Source: CAD feature listing. Evaluate the final solid. Frame: model axes, mm. Face numbers are marked on the shaded views. A direction names the side the tool comes from. Round coordinates to 2 decimals unless told otherwise and drop trailing zeros. Order: outer loops, then holes, each group sorted by start corner. A loop starts at its lowest first (then second) coordinate and runs counter-clockwise, first axis right, second up. Notation, with made-up numbers: (-31, 61.25) -> (4, 61.25) arc R22 cw to (4, 68.25) -> close; hole circle Ø6 at (-23, 38.25). An arc over 180 degrees is marked (long way). Answer as CSV lines item,"result".
from build123d import *

# Parameters (mm, degrees)
SKETCH1_W               = 40
SKETCH1_H               = 32
BOSS_EXTRUDE1_DEPTH     = 7
SKETCH2_R               = 14.05
CUT_EXTRUDE1_DEPTH      = 6
SKETCH3_R               = 8.7
CUT_EXTRUDE2_DEPTH      = 6
SKETCH4_R               = 1.5
CUT_EXTRUDE3_DEPTH      = 6
CHAMFER1_SIZE           = 1.45
CHAMFER1_SIZE_2         = 1.995753785
CUT_EXTRUDE4_DEPTH      = 39.379682143
CUT_EXTRUDE4_DEPTH_BACK = 39.379682143
SKETCH5_R               = 2
FILLET1_R               = 2
CUT_EXTRUDE5_START      = -5
SKETCH6_R               = 2.375
CUT_EXTRUDE5_DEPTH      = 5
CHAMFER2_SIZE           = 1


with BuildPart() as part:
    # Sketch1 → Boss-Extrude1 (new body)
    with BuildSketch(Plane.XY):
        Rectangle(SKETCH1_W, SKETCH1_H)
    extrude(amount=BOSS_EXTRUDE1_DEPTH)

    # Sketch2 → Cut-Extrude1 (cut)
    with BuildSketch(Plane(origin=(0, 0, 0), x_dir=(-1, 0, 0), z_dir=(0, 0, -1))):
        Circle(SKETCH2_R)
    extrude(amount=-CUT_EXTRUDE1_DEPTH, mode=Mode.SUBTRACT)

    # Sketch3 → Cut-Extrude2 (cut)
    with BuildSketch(Plane(origin=(0, 0, 6), x_dir=(-1, 0, 0), z_dir=(0, 0, -1))):
        Circle(SKETCH3_R)
    extrude(amount=-CUT_EXTRUDE2_DEPTH, mode=Mode.SUBTRACT)

    # Sketch4 → Cut-Extrude3 (cut)
    with BuildSketch(Plane(origin=(0, 0, 6), x_dir=(-1, 0, 0), z_dir=(0, 0, -1))):
        with Locations((0, 11)):
            Circle(SKETCH4_R)
        with Locations((11, 0)):
            Circle(SKETCH4_R)
        with Locations((0, -11)):
            Circle(SKETCH4_R)
        with Locations((-11, 0)):
            Circle(SKETCH4_R)
    extrude(amount=-CUT_EXTRUDE3_DEPTH, mode=Mode.SUBTRACT)

    # Chamfer1
    # the kernel refuses this chamfer: 1.995753785, 1.45 mm, written as the material it takes off along each edge
    with BuildSketch(Plane(origin=(0, -11, 7), x_dir=(-1, 0, 0), z_dir=(0, -1, 0))) as chamfer1_piece_1:
        Polygon((1.5 + CHAMFER1_SIZE, 0), (1.5, CHAMFER1_SIZE_2), (1.5, 0), align=None)
    revolve(axis=Axis((0, -11, 7), (0, 0, -1)), mode=Mode.SUBTRACT)
    with BuildSketch(Plane(origin=(-11, 0, 7), x_dir=(-1, 0, 0), z_dir=(0, -1, 0))) as chamfer1_piece_2:
        Polygon((1.5 + CHAMFER1_SIZE, 0), (1.5, CHAMFER1_SIZE_2), (1.5, 0), align=None)
    revolve(axis=Axis((-11, 0, 7), (0, 0, -1)), mode=Mode.SUBTRACT)
    with BuildSketch(Plane(origin=(11, 0, 7), x_dir=(-1, 0, 0), z_dir=(0, -1, 0))) as chamfer1_piece_3:
        Polygon((1.5 + CHAMFER1_SIZE, 0), (1.5, CHAMFER1_SIZE_2), (1.5, 0), align=None)
    revolve(axis=Axis((11, 0, 7), (0, 0, -1)), mode=Mode.SUBTRACT)
    with BuildSketch(Plane(origin=(0, 11, 7), x_dir=(-1, 0, 0), z_dir=(0, -1, 0))) as chamfer1_piece_4:
        Polygon((1.5 + CHAMFER1_SIZE, 0), (1.5, CHAMFER1_SIZE_2), (1.5, 0), align=None)
    revolve(axis=Axis((0, 11, 7), (0, 0, -1)), mode=Mode.SUBTRACT)

    # Sketch5 → Cut-Extrude4 (cut, two sides: drawn at the far end of the back side and taken through both)
    with BuildSketch(Plane(origin=(0, 16, 0), x_dir=(1, 0, 0), z_dir=(0, 1, 0)).offset(-CUT_EXTRUDE4_DEPTH_BACK)):
        with Locations(Location((-17, -4, 0), (0, 0, 270))):
            Circle(SKETCH5_R)
        with Locations(Location((17, -4, 0), (0, 0, 270))):
            Circle(SKETCH5_R)
    extrude(amount=CUT_EXTRUDE4_DEPTH + CUT_EXTRUDE4_DEPTH_BACK, mode=Mode.SUBTRACT)

    # Fillet1
    # the kernel refuses this fillet: 2 mm, written as the material it takes off along each edge
    with BuildSketch(Plane(origin=(20, -16, -5), x_dir=(0, 1, 0), z_dir=(0, 0, 1)), Plane(origin=(20, 16, -5), x_dir=(-1, 0, 0), z_dir=(0, 0, 1))) as fillet1_piece_1:
        with BuildLine():
            CenterArc((FILLET1_R, FILLET1_R), FILLET1_R, 180, 90)
            Line((0, FILLET1_R), (0, 0))
            Line((0, 0), (FILLET1_R, 0))
        make_face()
    extrude(amount=17, mode=Mode.SUBTRACT)
    with BuildSketch(Plane(origin=(-20, -16, -5), x_dir=(0, 1, 0), z_dir=(0, 0, 1)), Plane(origin=(-20, 16, -5), x_dir=(1, 0, 0), z_dir=(0, 0, 1))) as fillet1_piece_2:
        with BuildLine():
            CenterArc((FILLET1_R, -FILLET1_R), FILLET1_R, 90, 90)
            Line((0, -FILLET1_R), (0, 0))
            Line((0, 0), (FILLET1_R, 0))
        make_face()
    extrude(amount=17, mode=Mode.SUBTRACT)

    # Sketch6 → Cut-Extrude5 (cut)
    with BuildSketch(Plane(origin=(0, 16, 0), x_dir=(1, 0, 0), z_dir=(0, 1, 0)).offset(CUT_EXTRUDE5_START)):
        with Locations(Location((-17, -4, 0), (0, 0, 270))):
            Circle(SKETCH6_R)
        with Locations(Location((17, -4, 0), (0, 0, 270))):
            Circle(SKETCH6_R)
    cut_extrude5 = extrude(amount=-CUT_EXTRUDE5_DEPTH, mode=Mode.SUBTRACT)

    # Mirror1: Cut-Extrude5 across plane
    add(cut_extrude5.mirror(Plane.ZX), mode=Mode.SUBTRACT)

    # Chamfer2
    # the kernel refuses this chamfer: 1 mm, written as the material it takes off along each edge
    with BuildSketch(Plane(origin=(17, -16, 4), x_dir=(0.006283143965557505, 0, 0.9999802608561372), z_dir=(-0.9999802608561372, 0, 0.006283143965557505))) as chamfer2_piece_1:
        Polygon((2 + CHAMFER2_SIZE, 0), (2, CHAMFER2_SIZE), (2, 0), align=None)
    revolve(axis=Axis((17, -16, 4), (0, 1, 0)), revolution_arc=359.64, mode=Mode.SUBTRACT)
    with BuildSketch(Plane(origin=(-17, -16, 4), x_dir=(0, 0, 1), z_dir=(-1, 0, 0))) as chamfer2_piece_2:
        Polygon((2 + CHAMFER2_SIZE, 0), (2, CHAMFER2_SIZE), (2, 0), align=None)
    revolve(axis=Axis((-17, -16, 4), (0, 1, 0)), revolution_arc=359.64, mode=Mode.SUBTRACT)
    with BuildSketch(Plane(origin=(-17, 16, 4), x_dir=(0, 0, 1), z_dir=(-1, 0, 0))) as chamfer2_piece_3:
        Polygon((2 + CHAMFER2_SIZE, 0), (2, -CHAMFER2_SIZE), (2, 0), align=None)
    revolve(axis=Axis((-17, 16, 4), (0, 1, 0)), revolution_arc=359.64, mode=Mode.SUBTRACT)
    with BuildSketch(Plane(origin=(17, 16, 4), x_dir=(0.006283143965557505, 0, 0.9999802608561372), z_dir=(-0.9999802608561372, 0, 0.006283143965557505))) as chamfer2_piece_4:
        Polygon((2 + CHAMFER2_SIZE, 0), (2, -CHAMFER2_SIZE), (2, 0), align=None)
    revolve(axis=Axis((17, 16, 4), (0, 1, 0)), revolution_arc=359.64, mode=Mode.SUBTRACT)
    with BuildSketch(Plane(origin=(17, 16, 4), x_dir=(0, 0, 1), z_dir=(-1, 0, 0))) as chamfer2_piece_5:
        Polygon((2 + CHAMFER2_SIZE, 0), (2, -CHAMFER2_SIZE), (2, 0), align=None)
    revolve(axis=Axis((17, 16, 4), (0, 1, 0)), revolution_arc=251.029734773, mode=Mode.SUBTRACT)
    with BuildSketch(Plane(origin=(-17, 16, 4), x_dir=(0.9456874082674533, 0, -0.3250774151558165), z_dir=(0.3250774151558165, 0, 0.9456874082674533))) as chamfer2_piece_6:
        Polygon((2 + CHAMFER2_SIZE, 0), (2, -CHAMFER2_SIZE), (2, 0), align=None)
    revolve(axis=Axis((-17, 16, 4), (0, 1, 0)), revolution_arc=251.029734773, mode=Mode.SUBTRACT)
    with BuildSketch(Plane(origin=(-17, -16, 4), x_dir=(0.9456874082674562, 0, -0.3250774151558082), z_dir=(0.3250774151558082, 0, 0.9456874082674562))) as chamfer2_piece_7:
        Polygon((2 + CHAMFER2_SIZE, 0), (2, CHAMFER2_SIZE), (2, 0), align=None)
    revolve(axis=Axis((-17, -16, 4), (0, 1, 0)), revolution_arc=251.029734773, mode=Mode.SUBTRACT)
    with BuildSketch(Plane(origin=(17, -16, 4), x_dir=(0, 0, 1), z_dir=(-1, 0, 0))) as chamfer2_piece_8:
        Polygon((2 + CHAMFER2_SIZE, 0), (2, CHAMFER2_SIZE), (2, 0), align=None)
    revolve(axis=Axis((17, -16, 4), (0, 1, 0)), revolution_arc=251.029734773, mode=Mode.SUBTRACT)


solid = part.part
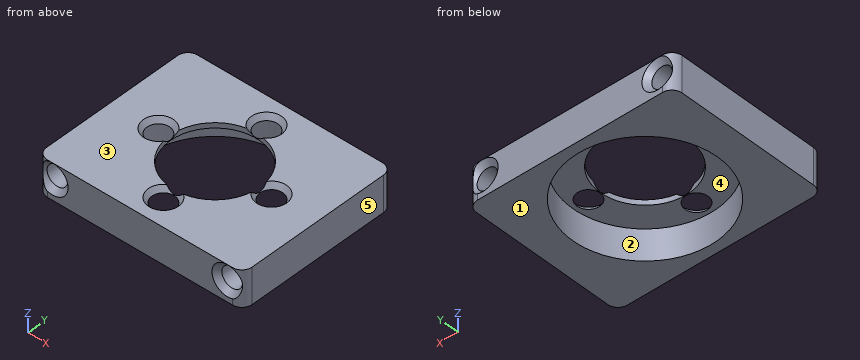
1. Section query B-B on z = 0.5. Return loops of the section in (x, y), and give its area (3 significant figures).
Results below:
outline,"(-20, -14) arc R2 ccw to (-18, -16) -> (18, -16) arc R2 ccw to (20, -14) -> (20, 14) arc R2 ccw to (18, 16) -> (-18, 16) arc R2 ccw to (-20, 14) -> close; hole circle Ø28.1 at (0, 0)"
area,"656 mm2"
2. Pin query (flat end, axial travel): pin 1 (3 mm diameter, centred on x = -17, z = 4, fed in from -Y); pin 2 (1.4 mm diameter, centred on x = 16, z = 3, fed in from -Y); pin 3 (2.5 mm diameter, centred on x = -18, z = 5, fed in from +Y). Return the tip coordinate at first contact, or that it passes through.
Results below:
pin 1,"through"
pin 2,"y = -15.11"
pin 3,"y = 15.66"
3. Line query: L1, parallel to Y at x = 0.5, z = 0.5; L2, parallel to X at y = -9.5, z = 5.25; L3, parallel to X at y = 7.25, z = 4 (3 decimals). Output: solid intervals per line, ascending. Write a range as [from, to].
Results below:
L1,"[-16, -14.04], [14.04, 16]"
L2,"[-20, -19.02], [-14.98, -10.35], [10.35, 14.98], [19.02, 20]"
L3,"[-20, -19.375], [-14.625, -12.035], [12.035, 14.625], [19.375, 20]"
4. Section query C-C on x = 0. Return loops of the section in (y, z), and give its area (3 significant figures).
Results below:
outline,"(-16, 0) -> (-14.05, 0) -> (-14.05, 6) -> (-13.22, 6) -> (-13.95, 7) -> (-16, 7) -> close; (-8.78, 6) -> (-8.7, 6) -> (-8.7, 6.11) -> close; (8.7, 6) -> (8.78, 6) -> (8.7, 6.11) -> close; (13.22, 6) -> (14.05, 6) -> (14.05, 0) -> (16, 0) -> (16, 7) -> (13.95, 7) -> close"
area,"28.2 mm2"
5. Reachability of the marked faces 1 and 2 from +Z, -Z, +X, -X, +Y, -Y: full face, straight path, thin tool, end or side. Return the list, or none.
Results below:
face 1,"-Z, +X, -X, +Y, -Y"
face 2,"-Z"
6. Section query D-D on y = -12. Give the number of separate pieces and of enclosed holes in the cut face, and give its area (3 significant figures).
Results below:
separate pieces,"2"
enclosed holes,"2"
area,"162 mm2"
7. Section query A-A on x = -5. Return loops of the section in (y, z), and give its area (3 significant figures).
Results below:
outline,"(-16, 0) -> (-13.13, 0) -> (-13.13, 6) -> (-7.12, 6) -> (-7.12, 7) -> (-16, 7) -> close; (7.12, 6) -> (13.13, 6) -> (13.13, 0) -> (16, 0) -> (16, 7) -> (7.12, 7) -> close"
area,"52.2 mm2"
8. Mould query, pull axis X, two halves, no side actions, for the marked faces 3, 4 and 5. Classes: released by +X, released by -X, zero draft, split by the parting line, or undercut.
Results below:
face 3,"zero draft"
face 4,"undercut"
face 5,"released by +X"
